Here's how the part is built. I have some questions about the finished solid (model axes, mm). A direction names the side the tool comes from. Coordinates: 2 decimals unless noted, no trailing zeros. Write each loop counter-clockwise with the first axis right and the second up, starting at its lowest first coordinate (ties: lowest second). Pieces come first, ordered by that corner, then holes.
from build123d import *

# Parameters (mm, degrees)
SKETCH010_W             = 100
SKETCH010_H             = 20
SKETCH010_R             = 2.6
PAD005_DEPTH            = 10
SKETCH012_W             = 23
SKETCH012_H             = 20
PAD003_DEPTH            = 22.5
POCKET005_DEPTH         = 10
SKETCH008_R             = 3.5
POCKET004_DEPTH         = 15
POCKET006_DEPTH         = 2
SKETCH013_W             = 5.5
SKETCH013_H             = 6
PAD004_DEPTH            = 10
FILLET002_R             = 2
FILLET003_R             = 1
SKETCH014_R             = 4.6
POCKET007_DEPTH         = 5
BODY001_PLACEMENT_ANGLE = 180


with BuildPart() as part:
    # Sketch010 → Pad005 (new body)
    with BuildSketch(Plane.XY):
        with Locations((50, 10)):
            Rectangle(SKETCH010_W, SKETCH010_H)
        with Locations((10, 10)):
            Circle(SKETCH010_R, mode=Mode.SUBTRACT)
    extrude(amount=PAD005_DEPTH)

    # Sketch012 (on Face7 of Pad005) → Pad003 (join)
    with BuildSketch(Plane.XY.offset(10)):
        with Locations((88.5, 10)):
            Rectangle(SKETCH012_W, SKETCH012_H)
    extrude(amount=PAD003_DEPTH)

    # Sketch009 (on Face11 of Pad003) → Pocket005 (cut)
    with BuildSketch(Plane.XY.offset(32.5)):
        with BuildLine():
            Line((97, 13), (97, 5))
            Line((80, 5), (97, 5))
            Line((80, 5), (80, 13))
            ThreePointArc((97, 13), (88.5, 14.984019), (80, 13))
        make_face()
    extrude(amount=-POCKET005_DEPTH, mode=Mode.SUBTRACT)

    # Sketch008 (on Face17 of Pocket005) → Pocket004 (cut)
    with BuildSketch(Plane.XY.offset(22.5)):
        with Locations((88.5, 10)):
            Circle(SKETCH008_R)
    extrude(amount=-POCKET004_DEPTH, mode=Mode.SUBTRACT)

    # Sketch011 (on Face5 of Pocket004) → Pocket006 (cut)
    with BuildSketch(Plane.XY.offset(10)):
        with BuildLine():
            Line((26.5, 12), (91.5, 12))
            Line((91.5, 12), (91.5, 8))
            Line((91.5, 8), (26.5, 8))
            ThreePointArc((26.5, 8), (24.732233, 7.267767), (24, 5.5))
            Line((24, 5.5), (24, 0))
            Line((24, 0), (20, 0))
            Line((20, 0), (20, 20))
            Line((20, 20), (24, 20))
            Line((24, 20), (24, 14.5))
            ThreePointArc((24, 14.5), (24.732233, 12.732233), (26.5, 12))
        make_face()
    extrude(amount=-POCKET006_DEPTH, mode=Mode.SUBTRACT)

    # Sketch013 → Pad004 (join)
    with BuildSketch(Plane.XY.offset(10)):
        with Locations((2.75, 10)):
            Rectangle(SKETCH013_W, SKETCH013_H)
        with Locations((17.25, 10)):
            Rectangle(SKETCH013_W, SKETCH013_H)
    extrude(amount=PAD004_DEPTH)

    # Fillet002
    fillet002_edges = [part.edges().sort_by_distance(p)[0] for p in [
        (77, 10, 32.5),
        (88.5, 0, 32.5),
        (88.5, 20, 32.5),
        (100, 10, 32.5),
        (100, 10, 0),
        (50, 20, 0),
        (0, 10, 0),
        (50, 0, 0),
        (77, 20, 21.25),
        (77, 0, 21.25),
        (100, 0, 21.25),
        (100, 20, 21.25),
        (0, 20, 5),
        (0, 0, 5),
    ]]
    fillet(fillet002_edges, radius=FILLET002_R)

    # Fillet003
    fillet003_edges = [part.edges().sort_by_distance(p)[0] for p in [
        (0, 18, 6),
        (50.5, 0, 10),
    ]]
    fillet(fillet003_edges, radius=FILLET003_R)

    # Sketch014 (on Face38 of Fillet003) → Pocket007 (cut)
    with BuildSketch(Plane(origin=(0, 0, 0), x_dir=(1, 0, 0), z_dir=(0, 0, -1))):
        with Locations((10, -10)):
            Circle(SKETCH014_R)
    extrude(amount=-POCKET007_DEPTH, mode=Mode.SUBTRACT)


with BuildPart() as part_1:
    # Body001 placement: moved
    add(part.part.moved(Location((0, 20, 320))).rotate(Axis((0, 20, 320), (1, 0, 0)), BODY001_PLACEMENT_ANGLE))


solid = part_1.part
1. If I drill on line 1 (X direction, y = 10, z = 303); line 2 (Y direction, x = 10, z = 312); line 3 (Y direction, x = 88.5, z = 304), over which ranges is the centre line in solid material (lowest first)?
2. Thinking about a two-plate mould opening in X: for faces 1 (the face through (99.4, 9.89, 288.07)), 2 (the face through (3, 7, 305)), 3 (the face through (88, 15, 292)), which applies, pulls with the +X half, pulls with the -X half, needs draft (parallel to the pull), parting line crosses it, or undercut?
3. I want a section at A-A (x = 10). List the corners of the cut face in (y, z) for me.
4. I want a section at D-D (x = 53). List the corners of the cut face in (y, z) for me, then the cut area to 3 significant figures.
5. I want a section at B-B (y = 10). State how many separate pieces and enclosed holes the cut face has, then the cut area to 3 significant figures.
6. I want a section at C-C (z = 296). List the corners of the cut face in (x, y) for me, then the cut area to 3 significant figures.
7. For pin 1 Ø1.5 at (y, z) = (9, 297.5) entering from -X; pin 2 Ø3 at (x, z) = (16, 303) entering from -Y; pin 3 Ø4.5 at (x, z) = (3, 303.5) entering from +Y, each with a flat end and sliding along its axis, tell me the tip position at first contact or that it passes through.
8. On a 3-axis mill with a long thin cutter (end or side, diameter ignored), from which of +Z, -Z, +X, -X, +Y, -Y can I reach the whole of each face in a straight line? I mean faces 4 (the face through (77.57, 0.6, 299.61)), 5 (the face through (77, 10, 300)), 6 (the face through (91.733, 11.341, 304.895)). Say none if no direction works.
Response values:
1. line 1: x = 0 to 5.5, 14.5 to 20, 77 to 85, 92 to 100
1. line 2: y = 0 to 7.4, 12.6 to 20
1. line 3: y = 0 to 6.5, 13.5 to 20
2. face 1: pulls with the +X half
2. face 2: needs draft
2. face 3: undercut
3. outline: (0, 310) - (7.4, 310) - (7.4, 315) - (5.4, 315) - (5.4, 320) - (2, 320) arc R2 ccw to (0, 318) - close; (12.6, 310) - (20, 310) - (20, 318) arc R2 ccw to (18, 320) - (14.6, 320) - (14.6, 315) - (12.6, 315) - close
4. outline: (0, 310) - (8, 310) - (8, 312) - (12, 312) - (12, 310) - (19, 310) arc R1 ccw to (20, 311) - (20, 318) arc R2 ccw to (18, 320) - (2, 320) arc R2 ccw to (0, 318) - close
4. area: 190 mm2
5. separate pieces: 3
5. enclosed holes: 0
5. area: 1,150 mm2
6. outline: (77, 2) arc R2 ccw to (79, 0) - (98, 0) arc R2 ccw to (100, 2) - (100, 18) arc R2 ccw to (98, 20) - (79, 20) arc R2 ccw to (77, 18) - close; hole (80, 7) arc R19.2 ccw to (97, 7) - (97, 15) - (80, 15) - close
6. area: 298 mm2
7. pin 1: stops at x = 77
7. pin 2: stops at y = 7
7. pin 3: stops at y = 13
8. face 4: -Z, -X, -Y
8. face 5: -Z, +Y, -Y
8. face 6: -Z
